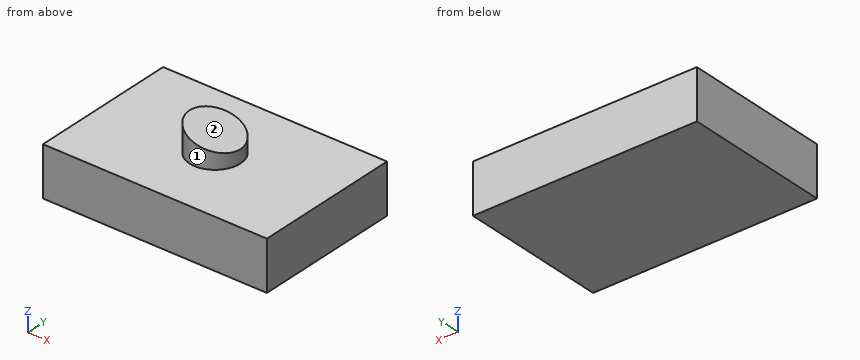
from build123d import *

# Parameters (mm, degrees)
F0_W     = 104.663714
F0_H     = 69.28701
F1_DEPTH = 23.114
F2_R     = 11.892204
F3_DEPTH = 18.034
F5_DEPTH = 25.4
F6_DEPTH = 25.4


with BuildPart() as f1:
    # F0 (on Top) → F1 (new body)
    with BuildSketch(Plane.XY):
        Rectangle(F0_W, F0_H)
    extrude(amount=F1_DEPTH)

    # F2 (on face) → F3 (join)
    with BuildSketch(Plane.XY.offset(23.114)):
        Circle(F2_R)
    extrude(amount=F3_DEPTH)

    # F4 (on Front) → F5 (cut)
    with BuildSketch(Plane.XZ):
        Polygon((20.987732, 43.441858), (-27.219897, 41.425567), (20.987732, 26.395051), align=None)
    extrude(amount=-F5_DEPTH, mode=Mode.SUBTRACT)

    # F4 (on Front) → F6 (cut)
    with BuildSketch(Plane.XZ):
        Polygon((20.987732, 43.441858), (-27.219897, 41.425567), (20.987732, 26.395051), align=None)
    extrude(amount=F6_DEPTH, mode=Mode.SUBTRACT)


solid = f1.part
Could you check a few things on this model? Use its own coordinates, in mm. Face numbers are marked on the shaded views. A direction names the side the tool comes from. Round coordinates to 2 decimals unless told otherwise and drop trailing zeros. Order: outer loops, then holes, each group sorted by start corner. A loop starts at its lowest first (then second) coordinate and runs counter-clockwise, first axis right, second up.
(1) Which directions (+Z, -Z, +X, -X, +Y, -Y) give clear straight access to the entire face, cutting with the end or side of a thin tool? Please do the marked faces 1 and 2.
Response values:
face 1: +Z
face 2: +Z, +X, +Y, -Y
(2) Imagine slicing it at A-A (y = 0). Write out the boundary of the cut face in (x, z).
Response values:
outline: (-52.33, 0) - (52.33, 0) - (52.33, 23.11) - (11.89, 23.11) - (11.89, 29.23) - (-11.89, 36.65) - (-11.89, 23.11) - (-52.33, 23.11) - close
(3) Imagine slicing it at B-B (x = 5.5). Write out the boundary of the cut face in (y, z), plus the area to 3 significant figures.
Response values:
outline: (-34.64, 0) - (34.64, 0) - (34.64, 23.11) - (10.54, 23.11) - (10.54, 31.22) - (-10.54, 31.22) - (-10.54, 23.11) - (-34.64, 23.11) - close
area: 1,770 mm2
(4) I'm going to push flat-ended pins straight in: pin 1 (3 mm diameter, centred on x = -27, y = -12.5, fed in from +Z); pin 2 (2 mm diameter, centred on y = -14.5, z = 29.5, fed in from +X); pin 3 (2 mm diameter, centred on x = 4, z = 29, fed in from +Y). Where does each tip first touch, or does it pass through?
Response values:
pin 1: stops at z = 23.11
pin 2: passes through
pin 3: stops at y = 11.51
(5) Imagine slicing it at D-D (x = -20.5). Write out the boundary of the cut face in (y, z), plus the area to 3 significant figures.
Response values:
outline: (-34.64, 0) - (34.64, 0) - (34.64, 23.11) - (-34.64, 23.11) - close
area: 1,600 mm2
(6) Imagine slicing it at C-C (y = 20). Write out the boundary of the cut face in (x, z).
Response values:
outline: (-52.33, 0) - (52.33, 0) - (52.33, 23.11) - (-52.33, 23.11) - close
(7) Please list where these lines run through material, in increasing order: line 1 along Z through (x, y) = (-35, -13.5); line 2 along Y through (x, z) = (-10, 26); line 3 along Y through (x, z) = (1, 26).
Response values:
line 1: z = 0 to 23.11
line 2: y = -6.44 to 6.44
line 3: y = -11.85 to 11.85
